Source: CAD feature listing. Evaluate the final solid. Frame: model axes, mm. Face numbers are marked on the shaded views. A direction names the side the tool comes from. Give positions to 0.01 mm unless a question says otherwise; leave off trailing zeros. Loops run counter-clockwise (first coordinate to the right, second up) from the corner with the lowest first, then second, coordinate; pieces in that order, holes last.
from build123d import *

# Parameters (mm, degrees)
BOSS_EXTRUDE1_DEPTH      = 20
BOSS_EXTRUDE1_DEPTH_BACK = 5
BOSS_EXTRUDE2_START      = -5
BOSS_EXTRUDE2_DEPTH      = 5
BOSS_EXTRUDE3_REACH      = 152.552
BOSS_EXTRUDE3_START      = -5


with BuildPart() as part:
    # Sketch1 → Boss-Extrude1 (new, two sides: drawn at the far end of the back side and taken through both)
    with BuildSketch(Plane.XY.offset(-BOSS_EXTRUDE1_DEPTH_BACK)):
        with BuildLine():
            Line((0, 25), (0, 17))
            ThreePointArc((0, 17), (-17, 0), (0, -17))
            Line((0, -17), (0, -25))
            ThreePointArc((0, -25), (-25, 0), (0, 25))
        make_face()
    extrude(amount=BOSS_EXTRUDE1_DEPTH + BOSS_EXTRUDE1_DEPTH_BACK)

    # Sketch2 → Boss-Extrude2 (add)
    with BuildSketch(Plane.XY.offset(BOSS_EXTRUDE2_START)):
        with BuildLine():
            Line((0, 25), (0, 77))
            Line((0, 77), (-65, 77))
            Line((-65, 77), (-65, 32.113081447))
            ThreePointArc((-65, 32.113081447), (-61.581037686, -38.262590053), (0, -72.5))
            Line((0, -72.5), (0, -25))
            ThreePointArc((0, -25), (-25, 0), (0, 25))
        make_face()
    extrude(amount=BOSS_EXTRUDE2_DEPTH)


with BuildPart() as body_2:
    # Mirror4: mirrored copy
    add(part.part.mirror(Plane.XY.offset(-40)))


with BuildPart() as part_1:
    add(part.part)

    # Sketch3 → Boss-Extrude3 (add, up to next)
    with BuildSketch(Plane(origin=(0, 0, -80), x_dir=(-1, 0, 0), z_dir=(0, 0, -1)).offset(BOSS_EXTRUDE3_START), mode=Mode.PRIVATE) as boss_extrude3_sk1:
        with BuildLine():
            Line((65, 77), (65, 32.113081447))
            ThreePointArc((65, 32.113081447), (61.581037686, -38.262590053), (0, -72.5))
            Line((0, -72.5), (0, -66.86))
            ThreePointArc((0, -66.86), (57.128742944, -34.735663656), (59.36, 30.767677845))
            Line((59.36, 30.767677845), (59.36, 77))
            Line((59.36, 77), (65, 77))
        make_face()
    boss_extrude3_tool1 = extrude(boss_extrude3_sk1.sketch, amount=-BOSS_EXTRUDE3_REACH, mode=Mode.PRIVATE) - part_1.part

    add(body_2.part)  # Boss-Extrude3 merges body 2
    add(boss_extrude3_tool1.solids().sort_by_distance((-61.02152, 53.883839, -75))[0])


solid = part_1.part
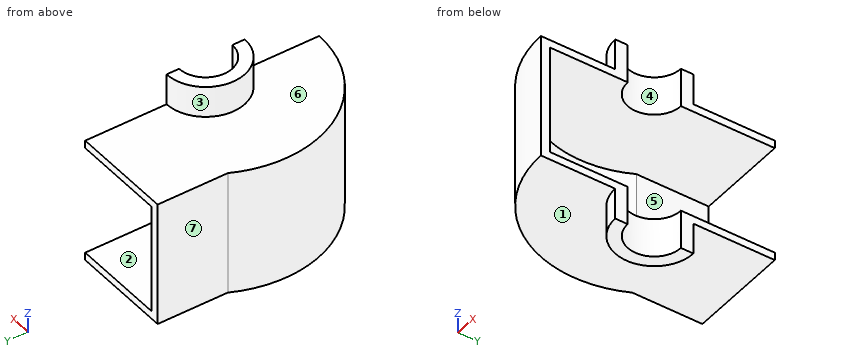
1) Ray query, probe 1 along Z at (x, y) = (-45.5, 36); probe 2 along Z at (x, y) = (-22.5, -1); probe 3 along X at (y, z) = (71.5, -63). Return the intervals inside material, ascending.
Checks:
probe 1: z = -80 to -75, -5 to 0
probe 2: z = -100 to -75, -5 to 20
probe 3: x = -65 to -59.36
2) Reachability of the marked faces 4, 5, 6 and 7 from +Z, -Z, +X, -X, +Y, -Y: full face, straight path, thin tool, end or side. Return the list, or none.
Checks:
face 4: +Z, -Z, +X
face 5: +X, +Y
face 6: +Z, -X
face 7: +Z, -Z, -X, +Y
3) Cut plane D-D (x = -63). Return loops of the section in (y, z), and give its area (3 significant figures).
Checks:
outline: (-35.88, -80) - (77, -80) - (77, 0) - (-35.88, 0) - close; hole (-22.39, -75) - (22.39, -75) - (22.39, -5) - (-22.39, -5) - close
area: 5,900 mm2
4) Contact query for flat-ended pins moving along their axis: P1, Ø3, axis at x = -23, z = -51, coming from the +Y side; P2, Ø1.5, axis at y = 16.5, z = -48, coming from the -X side; P3, Ø1.5, axis at x = -18, y = 61, coming from the -Z side. Output: stop coordinate, or through.
Checks:
P1: stops at y = -62.21
P2: stops at x = -70.77
P3: stops at z = -80
5) Cut plane B-B (z = -41). Return loops of the section in (x, y), and give its area (3 significant figures).
Checks:
outline: (-65, 32.11) arc R72.5 ccw to (0, -72.5) - (0, -66.86) arc R66.86 cw to (-59.36, 30.77) - (-59.36, 77) - (-65, 77) - close
area: 1,060 mm2
6) Pull-direction query (Z, two-part tool) for the marked faces 1, 2 and 3; classes: released by +Z, released by -Z, zero draft, split by the parting line, or undercut.
Checks:
face 1: released by -Z
face 2: undercut
face 3: zero draft
7) Cut plane C-C (x = -13.5). Return loops of the section in (y, z).
Checks:
outline: (-71.23, -80) - (-21.04, -80) - (-21.04, -100) - (-10.33, -100) - (-10.33, -75) - (-65.48, -75) - (-65.48, -5) - (-10.33, -5) - (-10.33, 20) - (-21.04, 20) - (-21.04, 0) - (-71.23, 0) - close; (10.33, -100) - (21.04, -100) - (21.04, -80) - (77, -80) - (77, -75) - (10.33, -75) - close; (10.33, -5) - (77, -5) - (77, 0) - (21.04, 0) - (21.04, 20) - (10.33, 20) - close
8) Cut plane A-A (y = 0). Return loops of the section in (x, z).
Checks:
outline: (-72.5, -80) - (-25, -80) - (-25, -100) - (-17, -100) - (-17, -75) - (-66.86, -75) - (-66.86, -5) - (-17, -5) - (-17, 20) - (-25, 20) - (-25, 0) - (-72.5, 0) - close
